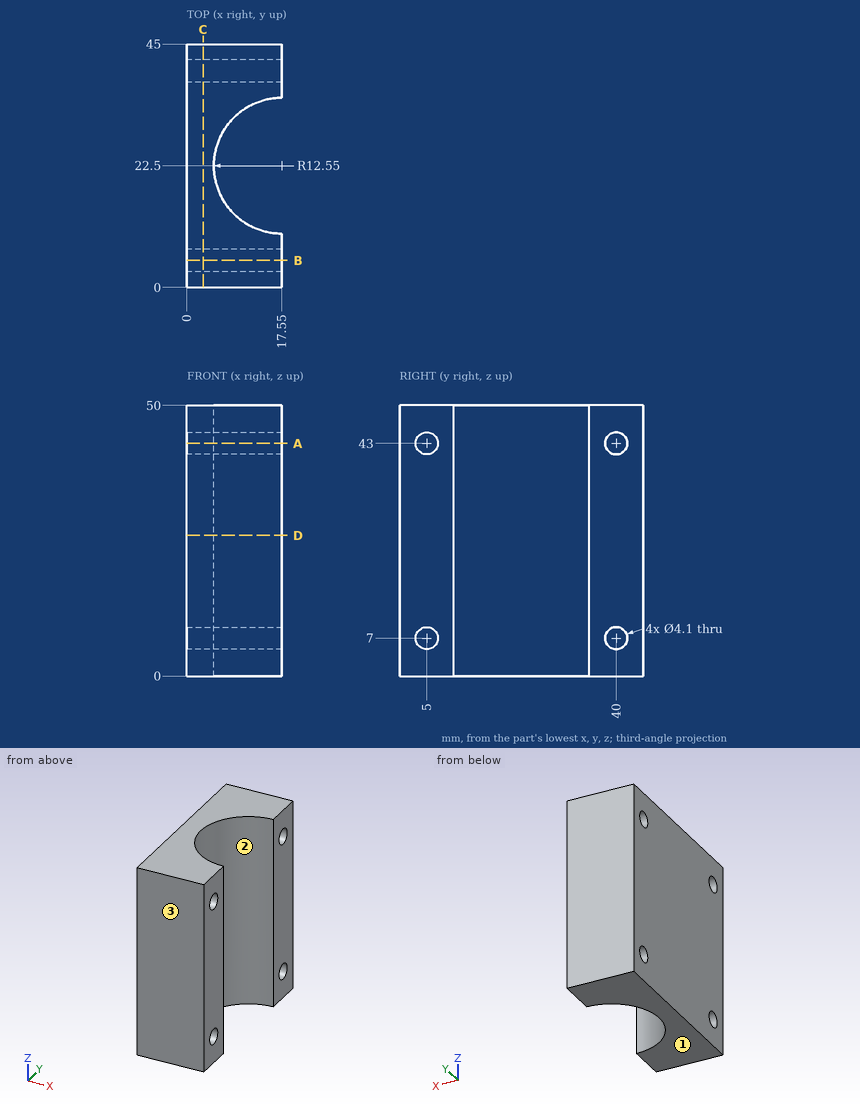
The figure shows three views and two pictorial views of one solid part (mm, origin at its lowest corner). Answer the questions. Coordinates: 2 decimals unless noted, no trailing zeros. Loops run counter-clockwise (first coordinate to the right, second up) from the corner with the lowest first, then second, coordinate; pieces in that order, holes last.
(1) Consider line 1 along Y through (x, z) = (4.75, 7); line 2 along Z through (x, y) = (11, 40); line 3 along Y through (x, z) = (10.5, 43). Determine where each line is inside the solid, lowest interval first.
Solution:
line 1: y = 0 to 2.95, 7.05 to 37.95, 42.05 to 45
line 2: z = 0 to 4.95, 9.05 to 40.95, 45.05 to 50
line 3: y = 0 to 2.95, 7.05 to 12.12, 32.88 to 37.95, 42.05 to 45
(2) The part is cut by section C-C (x = 3). Determine the outline of the cut face in (y, z), and give its area (3 significant figures).
Solution:
outline: (0, 0) - (45, 0) - (45, 50) - (0, 50) - close; hole circle Ø4.1 at (5, 7); hole circle Ø4.1 at (5, 43); hole circle Ø4.1 at (40, 7); hole circle Ø4.1 at (40, 43)
area: 2,200 mm2
(3) The part is cut by section A-A (z = 43). Determine the outline of the cut face in (x, y), and give its area (3 significant figures).
Solution:
outline: (0, 0) - (17.55, 0) - (17.55, 2.95) - (0, 2.95) - close; (0, 7.05) - (17.55, 7.05) - (17.55, 9.95) arc R12.55 cw to (17.55, 35.05) - (17.55, 37.95) - (0, 37.95) - close; (0, 42.05) - (17.55, 42.05) - (17.55, 45) - (0, 45) - close
area: 398 mm2
(4) The mould has two halves that part along Y. Classify the marked faces 1, 2 and 3: released by +Y, released by -Y, zero draft, split by the parting line, or undercut.
Solution:
face 1: zero draft
face 2: undercut
face 3: released by -Y
(5) The part is cut by section B-B (y = 5). Determine the outline of the cut face in (x, z).
Solution:
outline: (0, 0) - (17.55, 0) - (17.55, 4.95) - (0, 4.95) - close; (0, 9.05) - (17.55, 9.05) - (17.55, 40.95) - (0, 40.95) - close; (0, 45.05) - (17.55, 45.05) - (17.55, 50) - (0, 50) - close
(6) A flat-ended cylindrical pin translates along its axis: pin 1 Ø1.5 at (y, z) = (22, 8) entering from +X. Find the tip coordinate at first contact, or state that the pin passes through.
Solution:
pin 1: stops at x = 5.06
(7) The part is cut by section D-D (z = 26). Determine the outline of the cut face in (x, y).
Solution:
outline: (0, 0) - (17.55, 0) - (17.55, 9.95) arc R12.55 cw to (17.55, 35.05) - (17.55, 45) - (0, 45) - close
